```python
from build123d import *

# Parameters (mm, degrees)
SKETCH1_W           = 64
SKETCH1_H           = 90
BOSS_EXTRUDE1_DEPTH = 33
BOSS_EXTRUDE2_DEPTH = 24
SKETCH3_W           = 16
SKETCH3_H           = 92.520376572
CUT_EXTRUDE1_DEPTH  = 25
SKETCH6_W           = 16
SKETCH6_H           = 28
CUT_EXTRUDE3_DEPTH  = 45
SKETCH7_W           = 28
SKETCH7_H           = 14
CUT_EXTRUDE4_DEPTH  = 91


with BuildPart() as part:
    # Sketch1 → Boss-Extrude1 (new body)
    with BuildSketch(Plane(origin=(0, 0, 0), x_dir=(1, 0, 0), z_dir=(0, 1, 0))):
        Rectangle(SKETCH1_W, SKETCH1_H)
    extrude(amount=BOSS_EXTRUDE1_DEPTH)

    # Sketch2 → Boss-Extrude2 (add, symmetric)
    with BuildSketch(Plane(origin=(0, 0, 0), x_dir=(0, 0, -1), z_dir=(1, 0, 0))):
        with BuildLine():
            Line((45, 33), (-45, 33))
            Line((-45, 33), (-30, 70))
            Line((-30, 70), (-20, 70))
            ThreePointArc((-20, 70), (0, 50), (20, 70))
            Line((20, 70), (30, 70))
            Line((30, 70), (45, 33))
        make_face()
    extrude(amount=BOSS_EXTRUDE2_DEPTH, both=True)

    # Sketch3 → Cut-Extrude1 (cut)
    with BuildSketch(Plane(origin=(0, 70, 0), x_dir=(1, 0, 0), z_dir=(0, 1, 0))):
        Rectangle(SKETCH3_W, SKETCH3_H)
    extrude(amount=-CUT_EXTRUDE1_DEPTH, mode=Mode.SUBTRACT)

    # Sketch6 → Cut-Extrude3 (cut)
    with BuildSketch(Plane(origin=(0, 70, 0), x_dir=(1, 0, 0), z_dir=(0, 1, 0))):
        with Locations((24, 0)):
            Rectangle(SKETCH6_W, SKETCH6_H)
        with Locations((-24, 0)):
            Rectangle(SKETCH6_W, SKETCH6_H)
    extrude(amount=-CUT_EXTRUDE3_DEPTH, mode=Mode.SUBTRACT)

    # Sketch7 → Cut-Extrude4 (cut, through all)
    with BuildSketch(Plane.XY.offset(45)):
        with Locations((0, 7)):
            Rectangle(SKETCH7_W, SKETCH7_H)
    extrude(amount=-CUT_EXTRUDE4_DEPTH, mode=Mode.SUBTRACT)


solid = part.part
```
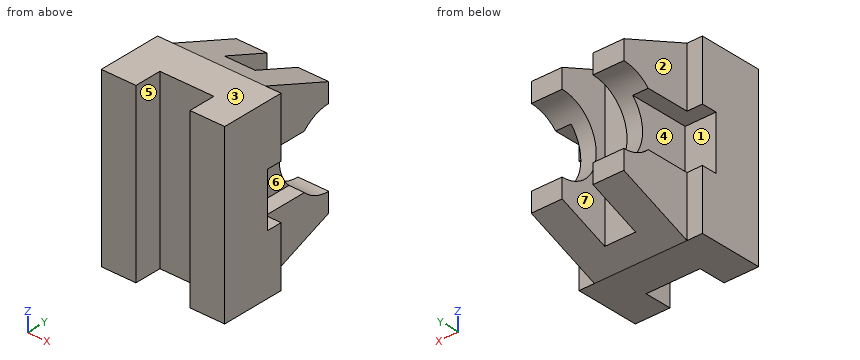
Source: CAD feature listing. Evaluate the final solid. Frame: model axes, mm. Face numbers are marked on the shaded views. A direction names the side the tool comes from. Give positions to 0.01 mm unless a question says otherwise; leave off trailing zeros. Write each loop counter-clockwise with the first axis right and the second up, starting at its lowest first coordinate (ties: lowest second). Pieces come first, ordered by that corner, then holes.
1. Section query B-B (y = 65). Return the cut outline in (x, z), then the cut area to 3 significant figures.
2. Section query C-C (z = -38.5). Return the cut outline in (x, y).
3. Pull-direction query (Z, two-part tool) for the marked faces 1, 2 and 3; classes: +Z half, -Z half, draft (parallel to the pull), parting line (faces both ways), or undercut.
4. Section query D-D (y = 51.5). Return the cut outline in (x, z).
5. First-contact query: pin 1 (4 mm diameter, centred on x = -16, y = 40.5, fed in from +Z); pin 2 (17.5 mm diameter, centred on x = 26.5, y = 46.5, fed in from +Z); pin 3 (1 mm diameter, centred on y = 30, z = 5, fed in from -X); pin 4 (12.5 mm diameter, centred on y = 62.5, z = -6, fed in from +X). Flat tips, straight axial feed; report the tip coordinate or a pass-through.
6. Section query A-A (x = 10.5). Return the cut outline in (y, z).
7. Access query for the marked faces 4, 5, 6 and 7. Directions: +Z, -Z, +X, -X, +Y, -Y. A direction counts if a zero-diameter tool reaches every point of the face in a straight line with its end or side. Return the directions, or none.
8. Material intervals for line 1 along X through (y, z) = (49.5, -17.5); line 2 along X through (y, z) = (49, 10); line 3 along Y through (x, z) = (7, 5.5), sorted ascending.
Output values:
1. outline: (-24, -32.03) - (-8, -32.03) - (-8, -19.36) - (-24, -19.36) - close; (-24, 19.36) - (-8, 19.36) - (-8, 32.03) - (-24, 32.03) - close; (8, -32.03) - (24, -32.03) - (24, -19.36) - (8, -19.36) - close; (8, 19.36) - (24, 19.36) - (24, 32.03) - (8, 32.03) - close
1. area: 810 mm2
2. outline: (-32, 0) - (-14, 0) - (-14, 14) - (14, 14) - (14, 0) - (32, 0) - (32, 33) - (24, 33) - (24, 49.03) - (8, 49.03) - (8, 45) - (-8, 45) - (-8, 49.03) - (-24, 49.03) - (-24, 33) - (-32, 33) - close
3. face 1: undercut
3. face 2: draft
3. face 3: +Z half
4. outline: (-24, -37.5) - (-8, -37.5) - (-8, -7.6) - (-16, -7.6) - (-16, -14) - (-24, -14) - close; (-24, 14) - (-16, 14) - (-16, 7.6) - (-8, 7.6) - (-8, 37.5) - (-24, 37.5) - close; (8, -37.5) - (24, -37.5) - (24, -14) - (16, -14) - (16, -7.6) - (8, -7.6) - close; (8, 7.6) - (16, 7.6) - (16, 14) - (24, 14) - (24, 37.5) - (8, 37.5) - close
5. pin 1: stops at z = 42.77
5. pin 2: stops at z = 42.93
5. pin 3: stops at x = -16
5. pin 4: passes through
6. outline: (14, -45) - (33, -45) - (70, -30) - (70, -20) arc R20 cw to (70, 20) - (70, 30) - (33, 45) - (14, 45) - close
7. face 4: -X, +Y
7. face 5: +Z, -Z, -Y
7. face 6: +X, +Y
7. face 7: +Z, -Z, +Y
8. line 1: x = -24 to -8, 8 to 24
8. line 2: x = -16 to -8, 8 to 16
8. line 3: y = 14 to 45
